Could you check a few things on this model? Use its own coordinates, in mm. Face numbers are marked on the shaded views. A direction names the side the tool comes from. Coordinates: 2 decimals unless noted, no trailing zeros. Loops run counter-clockwise (first coordinate to the right, second up) from the corner with the lowest first, then second, coordinate; pieces in that order, holes last. Notation, with made-up numbers: (-12, 21.5) -> (37, 21.5) arc R12 ccw to (37, 39.5) -> close; hole circle Ø3 at (51, 79.25). An arc over 180 degrees is marked (long way). One line per question, with ' | ' between items.
from build123d import *

# Parameters (mm, degrees)
SKETCH2_W               = 25
SKETCH2_H               = 6
BOSS_EXTRUDE2_DEPTH     = 45
BOSS_EXTRUDE3_DEPTH     = 35
SKETCH2_5_R             = 6
BOSS_EXTRUDE4_DEPTH     = 12
FILLET1_R               = 12
CUT_EXTRUDE1_DEPTH      = 87.890735985
CUT_EXTRUDE1_DEPTH_BACK = 87.890735985
SKETCH3_R               = 6


with BuildPart() as part:
    # Sketch2 → Boss-Extrude2 (new body)
    with BuildSketch(Plane.XY):
        with Locations((42.5, -9)):
            Rectangle(SKETCH2_W, SKETCH2_H)
        with Locations((-42.5, -9)):
            Rectangle(SKETCH2_W, SKETCH2_H)
        Polygon((55, -6), (55, 0), (11, 0), (-11, 0), (-55, 0), (-55, -6), (-30, -6), (30, -6), align=None)
    extrude(amount=BOSS_EXTRUDE2_DEPTH)

    # Sketch2_4 → Boss-Extrude3 (add)
    with BuildSketch(Plane.XY):
        with BuildLine():
            Line((0, 0), (11, 0))
            Line((11, 0), (20, 40))
            Line((20, 40), (25, 40))
            Line((25, 40), (25, 50))
            Line((25, 50), (15, 50))
            ThreePointArc((15, 50), (10.606601718, 39.393398282), (0, 35))
            Line((0, 35), (0, 0))
        make_face()
        with BuildLine():
            Line((-11, 0), (0, 0))
            Line((0, 0), (0, 35))
            ThreePointArc((0, 35), (-10.606601718, 39.393398282), (-15, 50))
            Line((-15, 50), (-25, 50))
            Line((-25, 50), (-25, 40))
            Line((-25, 40), (-20, 40))
            Line((-20, 40), (-11, 0))
        make_face()
    extrude(amount=BOSS_EXTRUDE3_DEPTH)

    # Sketch2_5 → Boss-Extrude4 (add)
    # profile 1 of 2: a face of its own
    with BuildSketch(Plane.XY):
        Polygon((11, 0), (55, 0), (55, 50), (25, 50), (25, 40), (20, 40), align=None)
        with Locations((43, 38)):
            Circle(SKETCH2_5_R, mode=Mode.SUBTRACT)
    # profile 2 of 2: a face of its own
    with BuildSketch(Plane.XY):
        Polygon((-55, 0), (-11, 0), (-20, 40), (-25, 40), (-25, 50), (-55, 50), align=None)
        with Locations((-43, 38)):
            Circle(SKETCH2_5_R, mode=Mode.SUBTRACT)
    extrude(amount=BOSS_EXTRUDE4_DEPTH)

    # Fillet1
    fillet1_edges = [part.edges().sort_by_distance(p)[0] for p in [
        (55, -6, 45),
        (-55, -6, 45),
        (55, 50, 6),
        (-55, 50, 6),
    ]]
    fillet(fillet1_edges, radius=FILLET1_R)

    # Sketch3 → Cut-Extrude1 (cut, two sides: drawn at the far end of the back side and taken through both)
    with BuildSketch(Plane(origin=(0, 0, 0), x_dir=(1, 0, 0), z_dir=(0, 1, 0)).offset(-CUT_EXTRUDE1_DEPTH_BACK)):
        with Locations(Location((-43, -33, 0), (0, 0, 270))):
            Circle(SKETCH3_R)
        with Locations(Location((43, -33, 0), (0, 0, 270))):
            Circle(SKETCH3_R)
    extrude(amount=CUT_EXTRUDE1_DEPTH + CUT_EXTRUDE1_DEPTH_BACK, mode=Mode.SUBTRACT)


solid = part.part
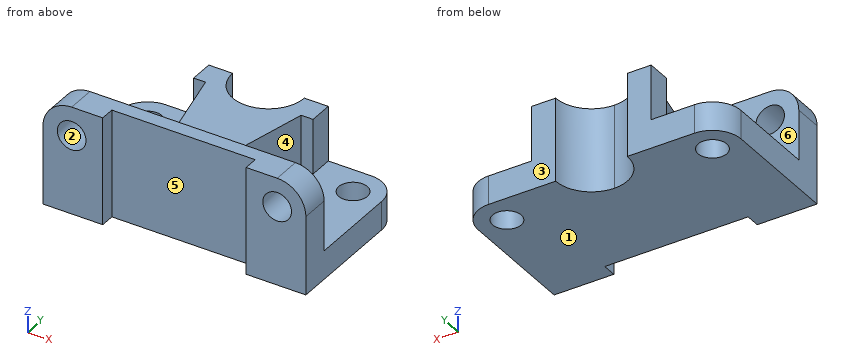
1) If we section it at D-D on x = 22.5: Please give me the cut outline in (y, z), and give its area (3 significant figures).
Data:
outline: (-6, 0) -> (50, 0) -> (50, 35) -> (40, 35) -> (40, 12) -> (0, 12) -> (0, 45) -> (-6, 45) -> close | area: 1,100 mm²
2) If we section it at A-A on y = -4: Please give me the cut outline in (x, z).
Data:
outline: (-55, 0) -> (55, 0) -> (55, 33) arc R12 ccw to (43, 45) -> (-43, 45) arc R12 ccw to (-55, 33) -> close; hole circle Ø12 at (-43, 33); hole circle Ø12 at (43, 33)
3) We'd pull the mould along Z, two halves only. Please class the marked faces 1, 2 and 3: pulls with the +Z half, pulls with the -Z half, needs draft (parallel to the pull), parting line crosses it, or undercut.
Data:
face 1: pulls with the -Z half | face 2: undercut | face 3: needs draft
4) If we section it at B-B on z = 10.5: Please give me the cut outline in (x, y), and give its area (3 significant figures).
Data:
outline: (-55, -12) -> (-30, -12) -> (-30, -6) -> (30, -6) -> (30, -12) -> (55, -12) -> (55, 38) arc R12 ccw to (43, 50) -> (15, 50) arc R15 cw to (-15, 50) -> (-43, 50) arc R12 ccw to (-55, 38) -> close; hole circle Ø12 at (-43, 38); hole circle Ø12 at (43, 38) | area: 5,820 mm²
5) On a 3-axis mill with a long thin cutter (end or side, diameter ignored), from which of +Z, -Z, +X, -X, +Y, -Y can I reach the whole of each face in a straight line? I mean the marked faces 4, 5 and 6. Say none if no direction works.
Data:
face 4: +Z, +X | face 5: +Z, -Z, -Y | face 6: +Z
6) I'm going to push flat-ended pins straight in: pin 1 Ø1.5 at (x, y) = (-9, 7) entering from +Z; pin 2 Ø7 at (x, z) = (43, 33) entering from +Y; pin 3 Ø19 at (x, z) = (-43, 33) entering from +Y; pin 4 Ø5 at (y, z) = (45, 20) entering from +X. Where does each tip first touch, or does it pass through?
Data:
pin 1: z = 35 | pin 2: through | pin 3: y = 0 | pin 4: x = 25
7) If we section it at C-C on z = 20: Please give me the cut outline in (x, y).
Data:
outline: (-55, -12) -> (-30, -12) -> (-30, -6) -> (30, -6) -> (30, -12) -> (55, -12) -> (55, 0) -> (11, 0) -> (20, 40) -> (25, 40) -> (25, 50) -> (15, 50) arc R15 cw to (-15, 50) -> (-25, 50) -> (-25, 40) -> (-20, 40) -> (-11, 0) -> (-55, 0) -> close
8) I need wall thicknesses on line 1 along X through (y, z) = (-5, 33); line 2 along X through (y, z) = (-6.25, 33); line 3 along Z through (x, y) = (43, -3). Which ranges of each line are inside material? Lowest first, please. Write a range as from..to.
Data:
line 1: -55..-49, -37..37, 49..55 | line 2: -55..-49, -37..-30, 30..37, 49..55 | line 3: 0..27, 39..45
